from build123d import *

# Parameters (mm, degrees)
SKETCH1_W           = 36
SKETCH1_H           = 40
SKETCH1_W_2         = 30
SKETCH1_H_2         = 35.5
BOSS_EXTRUDE1_DEPTH = 10
CUT_EXTRUDE2_REACH  = 46.989
FILLET1_R           = 3
FILLET2_R           = 1


with BuildPart() as part:
    # Sketch1 → Boss-Extrude1 (new body)
    with BuildSketch(Plane.XY):
        Rectangle(SKETCH1_W, SKETCH1_H)
        with Locations((0, -0.75)):
            Rectangle(SKETCH1_W_2, SKETCH1_H_2, mode=Mode.SUBTRACT)
    extrude(amount=BOSS_EXTRUDE1_DEPTH)

    # Sketch2 → Cut-Extrude2 (cut, up to next)
    with BuildSketch(Plane.XZ.offset(20), mode=Mode.PRIVATE) as cut_extrude2_sk1:
        with BuildLine():
            Line((-6, 10), (-2, 6.5))
            ThreePointArc((-2, 6.5), (0, 2.5), (2, 6.5))
            Line((2, 6.5), (6, 10))
            Line((6, 10), (-6, 10))
        make_face()
    cut_extrude2_tool1 = extrude(cut_extrude2_sk1.sketch, amount=-CUT_EXTRUDE2_REACH, mode=Mode.PRIVATE) & part.part
    add(cut_extrude2_tool1.solids().sort_by_distance((0, -20, 7.092656))[0], mode=Mode.SUBTRACT)

    # Fillet1
    fillet1_edges = [part.edges().sort_by_distance(p)[0] for p in [
        (-15, 17, 5),
        (-15, -18.5, 5),
        (15, -18.5, 5),
        (15, 17, 5),
    ]]
    fillet(fillet1_edges, radius=FILLET1_R)

    # Fillet2
    fillet2_edges = [part.edges().sort_by_distance(p)[0] for p in [
        (18, 0, 10),
        (0, 20, 10),
        (-18, 0, 10),
        (0, 20, 0),
        (18, 0, 0),
        (-18, 0, 0),
        (-18, 20, 5),
        (18, 20, 5),
        (18, -20, 5),
        (-18, -20, 5),
    ]]
    fillet(fillet2_edges, radius=FILLET2_R)


solid = part.part
Check sheet for the modelled part. Datum: model origin and axes. Units: mm. A direction names the side the tool comes from. Give positions to 0.01 mm unless a question says otherwise; leave off trailing zeros. Write each loop counter-clockwise with the first axis right and the second up, starting at its lowest first coordinate (ties: lowest second). Pieces come first, ordered by that corner, then holes. Notation, with made-up numbers: M 73.25,-0.5 L 96.25,-0.5 A8 ccw 96.25,6.5 Z; hole C -14,29.5 d9. An arc over 180 degrees is marked long. Use one line per item in the form item = value.
(1) Section check C-C on z = 5. Record the boundary of the cut face in (x, y).
Answer block:
outline = M -18,-19 A1 ccw -17,-20 L -2.5,-20 L -2.5,-18.5 L -12,-18.5 A3 cw -15,-15.5 L -15,14 A3 cw -12,17 L 12,17 A3 cw 15,14 L 15,-15.5 A3 cw 12,-18.5 L 2.5,-18.5 L 2.5,-20 L 17,-20 A1 ccw 18,-19 L 18,19 A1 ccw 17,20 L -17,20 A1 ccw -18,19 Z
(2) Section check D-D on x = 0. Record the boundary of the cut face in (y, z), plus the area to 3 significant figures.
Answer block:
outline = M -20,0 L -18.5,0 L -18.5,2.5 L -20,2.5 Z; M 17,0 L 19,0 A1 ccw 20,1 L 20,9 A1 ccw 19,10 L 17,10 Z
area = 33.3 mm2
(3) Tool access check on faces 5 (the cylindrical face through (17.699, -19.715, 5.07)), 6 (the cylindrical face through (-0.1, -19.3, 2.5)), 7 (the flat face through (-3, -18.5, 5)). Record the directions out of +Z, -Z, +X, -X, +Y, -Y that give a thin tool (end or side, any length) a straight path to the whole face; none if there is none.
Answer block:
face_5 = +Z, -Z, +X, -Y
face_6 = -Y
face_7 = +Z, -Z
(4) Material ranges on line 1 along Y through (x, z) = (10.5, 7.5); line 2 along X through (y, z) = (-1.5, 2); line 3 along X through (y, z) = (-18.9, 5), recorded low to high.
Answer block:
line_1 = -20 to -18.5, 17 to 20
line_2 = -18 to -15, 15 to 18
line_3 = -18 to -2.5, 2.5 to 18
(5) Section check A-A on y = -6.5. Record the boundary of the cut face in (x, z), plus the area to 3 significant figures.
Answer block:
outline = M -18,1 A1 ccw -17,0 L -15,0 L -15,10 L -17,10 A1 ccw -18,9 Z; M 15,0 L 17,0 A1 ccw 18,1 L 18,9 A1 ccw 17,10 L 15,10 Z
area = 59.1 mm2
(6) Section check B-B on x = -8. Record the boundary of the cut face in (y, z).
Answer block:
outline = M -20,0 L -18.5,0 L -18.5,10 L -20,10 Z; M 17,0 L 19,0 A1 ccw 20,1 L 20,9 A1 ccw 19,10 L 17,10 Z
(7) Draft check along X on faces 1 (the flat face through (0, -20, 2)), 2 (the cylindrical face through (-17.699, -0.227, 0.285)), 3 (the cylindrical face through (17.699, 19.715, 5.056)), 4 (the flat face through (-15, -1, 5)). Enter one of: pulls with the +X half, pulls with the -X half, needs draft (parallel to the pull), parting line crosses it, or undercut.
Answer block:
face_1 = needs draft
face_2 = pulls with the -X half
face_3 = pulls with the +X half
face_4 = undercut
